Source: CAD feature listing. Evaluate the final solid. Frame: model axes, mm. Face numbers are marked on the shaded views. A direction names the side the tool comes from. Coordinates: 2 decimals unless noted, no trailing zeros. Write each loop counter-clockwise with the first axis right and the second up, starting at its lowest first coordinate (ties: lowest second). Pieces come first, ordered by that corner, then holes. Notation, with made-up numbers: (73.5, 32.5) -> (89.5, 32.5) arc R11 cw to (89.5, 38.5) -> close; hole circle Ø11 at (-28, 72). An arc over 180 degrees is marked (long way). Write item = value, one per line.
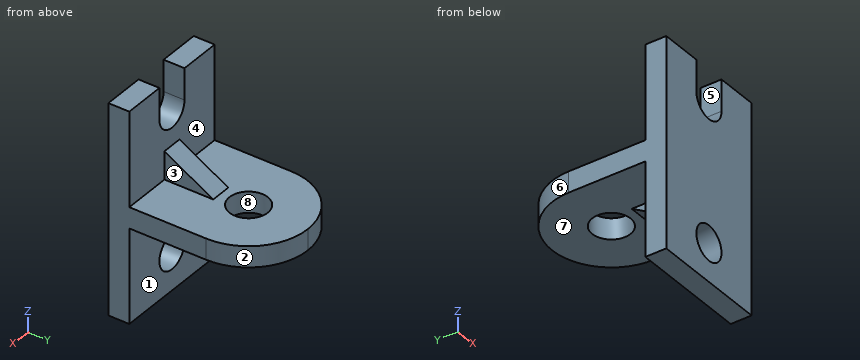
from build123d import *

# Parameters (mm, degrees)
EXTRUDE_1_DEPTH      = 17
EXTRUDE_1_DEPTH_BACK = 17
SKETCH_1_W           = 6
SKETCH_1_H           = 39
FILLET_1_R           = 17
SKETCH_2_R           = 5.5
CUT_EXTRUDE_1_DEPTH  = 46.036096634
EXTRUDE_2_DEPTH      = 3
EXTRUDE_2_DEPTH_BACK = 3
SKETCH_3_R           = 5
CUT_EXTRUDE_2_DEPTH  = 53.057660339


with BuildPart() as part:
    # Эскиз1 → Бобышка-Вытянуть1 (new, two sides: drawn at the far end of the back side and taken through both)
    with BuildSketch(Plane(origin=(0, 0, 0), x_dir=(0, 0, -1), z_dir=(1, 0, 0)).offset(-EXTRUDE_1_DEPTH_BACK)):
        Rectangle(SKETCH_1_W, SKETCH_1_H)
        Polygon((-3, -19.5), (-11, -19.5), (-30, -19.5), (-30, -25.5), (30, -25.5), (30, -19.5), (11, -19.5), (3, -19.5), align=None)
    extrude(amount=EXTRUDE_1_DEPTH + EXTRUDE_1_DEPTH_BACK)

    # Скругление1
    fillet_1_edges = [part.edges().sort_by_distance(p)[0] for p in [
        (17, 19.5, 0),
        (-17, 19.5, 0),
    ]]
    fillet(fillet_1_edges, radius=FILLET_1_R - 0.0001)  # a hair under: the kernel refuses the full size

    # Эскиз2 → Вырез-Вытянуть1 (cut, through all)
    with BuildSketch(Plane.XY.offset(3)):
        with Locations((0, 2.5)):
            Circle(SKETCH_2_R)
    extrude(amount=-CUT_EXTRUDE_1_DEPTH, mode=Mode.SUBTRACT)

    # Эскиз1<3> → Бобышка-Вытянуть2 (add, two sides: drawn at the far end of the back side and taken through both)
    with BuildSketch(Plane(origin=(0, 0, 0), x_dir=(0, 0, -1), z_dir=(1, 0, 0)).offset(-EXTRUDE_2_DEPTH_BACK)):
        Polygon((-3, -5.5), (-11, -19.5), (-3, -19.5), align=None)
        Polygon((3, -5.5), (3, -19.5), (11, -19.5), align=None)
    extrude(amount=EXTRUDE_2_DEPTH + EXTRUDE_2_DEPTH_BACK)

    # Эскиз3 → Вырез-Вытянуть2 (cut, through all)
    with BuildSketch(Plane(origin=(0, -19.5, 0), x_dir=(1, 0, 0), z_dir=(0, 1, 0))):
        with Locations(Location((0, 19, 0), (0, 0, 270))):
            Circle(SKETCH_3_R)
        with Locations((0, -21)):
            Circle(SKETCH_3_R)
        with BuildLine():
            ThreePointArc((5, -21), (0, -26), (-5, -21))
            Line((-5, -21), (-5, -30))
            Line((-5, -30), (5, -30))
            Line((5, -30), (5, -21))
        make_face()
    extrude(amount=-CUT_EXTRUDE_2_DEPTH, mode=Mode.SUBTRACT)


solid = part.part
1) Cut plane C-C, the plane y = 5. Output: boundary loops of the cut face in (x, z).
Answer block:
outline = (-16.82, -3) -> (-4.9, -3) -> (-4.9, 3) -> (-16.82, 3) -> close; (4.9, -3) -> (16.82, -3) -> (16.82, 3) -> (4.9, 3) -> close
2) Cut plane B-B, the plane z = 9. Output: boundary loops of the cut face in (x, y).
Answer block:
outline = (-17, -25.5) -> (17, -25.5) -> (17, -19.5) -> (3, -19.5) -> (3, -16) -> (-3, -16) -> (-3, -19.5) -> (-17, -19.5) -> close
3) Pull-direction query (Y, two-part tool) for the marked faces 6, 7 and 8; classes: +Y half, -Y half, draft (parallel to the pull), parting line (faces both ways), or undercut.
Answer block:
face_6 = +Y half
face_7 = draft
face_8 = undercut
4) Reachability of the marked faces 1, 2, 3, 4 and 5 from +Z, -Z, +X, -X, +Y, -Y: full face, straight path, thin tool, end or side. Return the list, or none.
Answer block:
face_1 = -Z, +Y
face_2 = +Z, -Z, +X, +Y
face_3 = +Z, +X, +Y
face_4 = +Z, +Y
face_5 = +Z, +Y, -Y
5) Cut plane D-D, the plane y = -15. Output: boundary loops of the cut face in (x, z), and give its area (3 significant figures).
Answer block:
outline = (-17, -3) -> (-3, -3) -> (-3, -8.43) -> (3, -8.43) -> (3, -3) -> (17, -3) -> (17, 3) -> (3, 3) -> (3, 8.43) -> (-3, 8.43) -> (-3, 3) -> (-17, 3) -> close
area = 269 mm2
6) Material intervals for probe 1 along X at (y, z) = (-21.7, -19); probe 2 along Y at (x, z) = (0, 0); probe 3 along Y at (x, z) = (-9.5, -12.5), sorted ascending. Write a range as [from, to].
Answer block:
probe_1 = [-17, -5], [5, 17]
probe_2 = [-25.5, -3], [8, 19.5]
probe_3 = [-25.5, -19.5]
7) Cut plane A-A, the plane z = -23. Output: boundary loops of the cut face in (x, y).
Answer block:
outline = (-17, -25.5) -> (-3, -25.5) -> (-3, -19.5) -> (-17, -19.5) -> close; (3, -25.5) -> (17, -25.5) -> (17, -19.5) -> (3, -19.5) -> close
8) First-contact query: pin 1 Ø17 at (x, y) = (2.5, -0.5) entering from -Z; pin 2 Ø4 at (x, z) = (-4, 6) entering from +Y; pin 3 Ø10 at (x, y) = (0, 6.5) entering from -Z; pin 4 Ø8 at (x, z) = (0, -19) entering from -Y. Flat tips, straight axial feed; report the tip coordinate or a pass-through.
Answer block:
pin_1 = -5
pin_2 = -7.72
pin_3 = -3
pin_4 = through
